from build123d import *

# Parameters (mm, degrees)
F0_W     = 117.5
F0_H     = 71.5
F1_DEPTH = 7


with BuildPart() as f1:
    # F0 (on Top) → F1 (new body)
    with BuildSketch(Plane.XY):
        Rectangle(F0_W, F0_H)
        with BuildLine():
            Line((20.634694, -6.987499), (0, -31.555828))
            Line((0, -31.555828), (-20.634694, -6.987499))
            ThreePointArc((-20.634694, -6.987499), (-17.241509, 11.252086), (0, 4.401793))
            ThreePointArc((0, 4.401793), (17.241509, 11.252086), (20.634694, -6.987499))
        make_face(mode=Mode.SUBTRACT)
    extrude(amount=F1_DEPTH)


solid = f1.part
Verification items for the finished model (mm, model axes). A direction names the side the tool comes from. Coordinates: 2 decimals unless noted, no trailing zeros. Order: outer loops, then holes, each group sorted by start corner. A loop starts at its lowest first (then second) coordinate and runs counter-clockwise, first axis right, second up. Notation, with made-up numbers: (7, -18) -> (49, -18) arc R20 cw to (49, 3) -> close; hole circle Ø4 at (-10, 71.5). An arc over 180 degrees is marked (long way). Use CSV: the item, a comma, the result in double quotes. Start each with the question number.
Q1. Thickness scan on line 1 along X through (y, z) = (6.5, 1.5); line 2 along Y through (x, z) = (-6, 2.75); line 3 along X through (y, z) = (8, 6). Record the ranges inside material, lowest first.
Q2. Draft check along X on faces 3 (the flat face through (58.75, -1, 3)), 4 (the flat face through (10.46, -19.1, 3.45)), 5 (the flat face through (-1, -35.75, 3)), 6 (the flat face through (-58.75, -1, 3)). Enter one of: +X half, -X half, draft (parallel to the pull), parting line (faces both ways), or undercut.
Q3. Section check D-D, the plane z = 4.75. Record the cut outline in (x, y).
Q4. Section check B-B, the plane x = 13. Record the cut outline in (y, z), and give its area (3 significant figures).
Q5. Section check C-C, the plane y = 7. Record the cut outline in (x, z).
Q6. Tool access check on faces 1 (the flat face through (-10.173, -19.444, 3.451)), 2 (the flat face through (-1, 8, 7)). Record the directions out of +Z, -Z, +X, -X, +Y, -Y that give a thin tool (end or side, any length) a straight path to the whole face; none if there is none.
Q7. Section check A-A, the plane y = -29.5. Record the cut outline in (x, z), and give its area (3 significant figures).
Q8. Depth check by flat-ended pin: P1, Ø14.5, axis at x = -11.44, y = 0.74, coming from the -Z side. Enter the tip coordinate at first touch or a pass-through.
Returned:
1,line 1,"x = -58.75 to -21.98, -0.9 to 0.9, 21.98 to 58.75"
1,line 2,"y = -35.75 to -24.41, 11.45 to 35.75"
1,line 3,"x = -58.75 to -21, -1.87 to 1.87, 21 to 58.75"
2,face 3,"+X half"
2,face 4,"undercut"
2,face 5,"draft"
2,face 6,"-X half"
3,outline,"(-58.75, -35.75) -> (58.75, -35.75) -> (58.75, 35.75) -> (-58.75, 35.75) -> close; hole (-20.63, -6.99) -> (0, -31.56) -> (20.63, -6.99) arc R12.01 ccw (long way) to (0, 4.4) arc R12.01 ccw (long way) to start"
4,outline,"(-35.75, 0) -> (-16.08, 0) -> (-16.08, 7) -> (-35.75, 7) -> close; (12.65, 0) -> (35.75, 0) -> (35.75, 7) -> (12.65, 7) -> close"
4,area,"299 mm^2"
5,outline,"(-58.75, 0) -> (-21.69, 0) -> (-21.69, 7) -> (-58.75, 7) -> close; (-1.19, 0) -> (1.19, 0) -> (1.19, 7) -> (-1.19, 7) -> close; (21.69, 0) -> (58.75, 0) -> (58.75, 7) -> (21.69, 7) -> close"
6,face 1,"+Z, -Z"
6,face 2,"+Z, +X, -X, +Y, -Y"
7,outline,"(-58.75, 0) -> (-1.73, 0) -> (-1.73, 7) -> (-58.75, 7) -> close; (1.73, 0) -> (58.75, 0) -> (58.75, 7) -> (1.73, 7) -> close"
7,area,"798 mm^2"
8,P1,"passes through"
